Check sheet for the modelled part. Datum: model origin and axes. Units: mm. Give positions to 0.01 mm unless a question says otherwise; leave off trailing zeros. Loops run counter-clockwise (first coordinate to the right, second up) from the corner with the lowest first, then second, coordinate; pieces in that order, holes last. Notation, with made-up numbers: (87, 81.5) - (146, 81.5) arc R13 cw to (146, 101.5) - close; hole circle Ø8 at (75.25, 21.5). An arc over 180 degrees is marked (long way). Answer in a Markdown table with one row per item. Add a question column.
(1) Sectioned sample at B-B on z = 30. Enter the section's corners in (x, y).
(2) Thickness scan on L1, parallel to X at y = 0.25, z = 31. Record the ranges inside material, lowest first.
(3) Go/stop test with flat-tipped pins: P1, Ø1, axis at y = 0, z = -5.5, coming from the +X side; P2, Ø1, axis at y = 0, z = -37, coming from the -X side. Record where each tip stops, or that it passes through.
(4) Sectioned sample at A-A on y = -1.75. Enter the section's corners in (x, z), then the cut area to 3 significant figures.
from build123d import *

# Parameters (mm, degrees)
ESQUISSE1_W             = 140
ESQUISSE1_H             = 7
BOSS_EXTRU_1_DEPTH      = 329
ESQUISSE2_W             = 303
ESQUISSE2_H             = 244.18
BOSS_EXTRU_2_DEPTH      = 7
ESQUISSE3_W             = 13
ESQUISSE3_H             = 110
ENL_V_MAT_EXTRU_1_DEPTH = 96
ENL_V_MAT_EXTRU_2_DEPTH = 96


with BuildPart() as part:
    # Esquisse1 → Boss.-Extru.1 (new body)
    with BuildSketch(Plane(origin=(0, 0, 0), x_dir=(0, 0, -1), z_dir=(1, 0, 0))):
        Rectangle(ESQUISSE1_W, ESQUISSE1_H)
    extrude(amount=BOSS_EXTRU_1_DEPTH)

    # Esquisse2 → Boss.-Extru.2 (add)
    with BuildSketch(Plane(origin=(0, 3.5, 0), x_dir=(1, 0, 0), z_dir=(0, 1, 0))):
        with Locations((164.5, 0)):
            Rectangle(ESQUISSE2_W, ESQUISSE2_H)
    extrude(amount=-BOSS_EXTRU_2_DEPTH)

    # Esquisse3 → Enlèv. mat.-Extru.1 (cut)
    with BuildSketch(Plane(origin=(0, 3.5, 0), x_dir=(1, 0, 0), z_dir=(0, 1, 0))):
        with Locations((6.5, 0)):
            Rectangle(ESQUISSE3_W, ESQUISSE3_H)
        with Locations((322.5, 0)):
            Rectangle(ESQUISSE3_W, ESQUISSE3_H)
    extrude(amount=-ENL_V_MAT_EXTRU_1_DEPTH, mode=Mode.SUBTRACT)

    # Esquisse4 → Enlèv. mat.-Extru.2 (cut)
    with BuildSketch(Plane(origin=(0, 3.5, 0), x_dir=(1, 0, 0), z_dir=(0, 1, 0))):
        Polygon((13, 70), (316, 70), (318.765325252, 132.447128924), (0, 132.447128924), align=None)
        Polygon((13, -70), (316, -70), (321.257609936, -130.666925578), (0, -142.41626766), align=None)
    extrude(amount=-ENL_V_MAT_EXTRU_2_DEPTH, mode=Mode.SUBTRACT)


solid = part.part
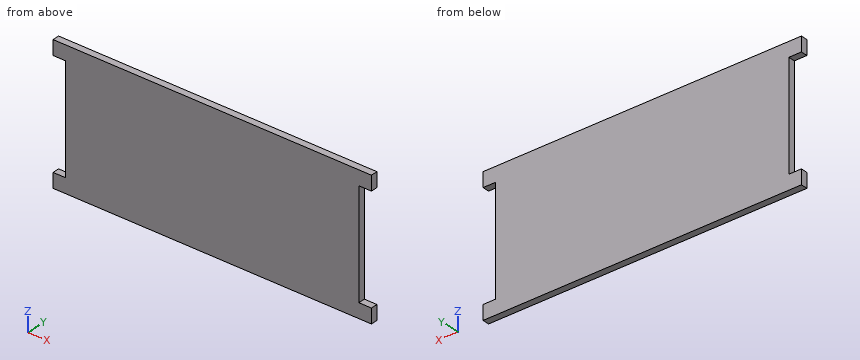
Reply:
| question | item | result |
|---|---|---|
| 1 | outline | (13, -3.5) - (316, -3.5) - (316, 3.5) - (13, 3.5) - close |
| 2 | L1 | 13 to 316 |
| 3 | P1 | x = 316 |
| 3 | P2 | x = 13 |
| 4 | outline | (0, -70) - (329, -70) - (329, -55) - (316, -55) - (316, 55) - (329, 55) - (329, 70) - (0, 70) - (0, 55) - (13, 55) - (13, -55) - (0, -55) - close |
| 4 | area | 43,200 mm^2 |
